Read the model definition and answer for the solid it produces. Units are mm, in the model's axes. A direction names the side the tool comes from. Give positions to 0.01 mm unless a question says otherwise; leave off trailing zeros. Write each loop counter-clockwise with the first axis right and the second up, starting at its lowest first coordinate (ties: lowest second). Pieces come first, ordered by that corner, then holes. Notation, with made-up numbers: M 54.25,-29 L 110.25,-29 A20 cw 110.25,-23 Z; hole C -24,30.5 d3. An arc over 180 degrees is marked long. Put each result on its own line as item: value.
from build123d import *

# Parameters (mm, degrees)
SKETCH1_W           = 230.12
SKETCH1_H           = 50.974909876
SKETCH1_R           = 7.058173785
BOSS_EXTRUDE1_DEPTH = 2
SKETCH2_R           = 10
BOSS_EXTRUDE2_DEPTH = 100
BOSS_EXTRUDE3_DEPTH = 10
FILLET1_R           = 5


with BuildPart() as part:
    # Sketch1 → Boss-Extrude1 (new body)
    with BuildSketch(Plane(origin=(0, 0, 0), x_dir=(1, 0, 0), z_dir=(0, 1, 0))):
        Rectangle(SKETCH1_W, SKETCH1_H)
        with Locations(Location((-95.06, 0, 0), (0, 0, 270))):
            Circle(SKETCH1_R, mode=Mode.SUBTRACT)
        with Locations(Location((95.06, 0, 0), (0, 0, 270))):
            Circle(SKETCH1_R, mode=Mode.SUBTRACT)
    extrude(amount=BOSS_EXTRUDE1_DEPTH)

    # Sketch2 → Boss-Extrude2 (add)
    with BuildSketch(Plane(origin=(0, 2, 0), x_dir=(1, 0, 0), z_dir=(0, 1, 0))):
        with Locations(Location((0, 0, 0), (0, 0, 270))):
            Circle(SKETCH2_R)
    extrude(amount=-BOSS_EXTRUDE2_DEPTH)

    # Sketch3 → Boss-Extrude3 (add)
    with BuildSketch(Plane(origin=(0, -98, 0), x_dir=(-1, 0, 0), z_dir=(0, -1, 0))):
        Polygon((15, 15), (30, 15), (30, -15), (15, -15), (15, -30), (-15, -30), (-15, -15), (-30, -15), (-30, 15), (-15, 15), (-15, 30), (15, 30), align=None)
    extrude(amount=BOSS_EXTRUDE3_DEPTH)

    # Fillet1
    fillet1_edges = [part.edges().sort_by_distance(p)[0] for p in [
        (0, 0, -10),
        (0, -98, -10),
    ]]
    fillet(fillet1_edges, radius=FILLET1_R)


solid = part.part
(1) Section A-A on z = 19.5 is taken. Determine the outline of the cut face in (x, y), and give its area (3 significant figures).
Result:
outline: M -115.06,0 L 115.06,0 L 115.06,2 L -115.06,2 Z; M -15,-108 L 15,-108 L 15,-98 L -15,-98 Z
area: 760 mm²
(2) Which of the six approach directions +Z, -Z, +X, -X, +Y, -Y give full straight-line access (tool end or side, diameter ignored) to faces 1 (the face through (-30, -103, 0)), 2 (the face through (-7, -98, -14)), 3 (the face through (23, -103, -15)), 4 (the face through (30, -103, 0)), 5 (the face through (22, -103, 15))?
Result:
face 1: +Z, -Z, -X, -Y
face 2: none
face 3: -Z, +X, -Y
face 4: +Z, -Z, +X, -Y
face 5: +Z, +X, -Y
(3) Section C-C on x = 95.06 is taken. Determine the outline of the cut face in (y, z).
Result:
outline: M 0,-25.49 L 2,-25.49 L 2,-7.06 L 0,-7.06 Z; M 0,7.06 L 2,7.06 L 2,25.49 L 0,25.49 Z
(4) Section D-D on x = 0 is taken. Determine the outline of the cut face in (y, z), and give its area (3 significant figures).
Result:
outline: M -108,-30 L -98,-30 L -98,-15 A5 cw -93,-10 L -5,-10 A5 cw 0,-15 L 0,-25.49 L 2,-25.49 L 2,25.49 L 0,25.49 L 0,15 A5 cw -5,10 L -93,10 A5 cw -98,15 L -98,30 L -108,30 Z
area: 2,680 mm²
(5) Given pin 1 Ø3 at (x, y) = (20.5, -103.5) entering from +Z; pin 2 Ø5 at (x, z) = (-53.5, -8) entering from -Y; pin 3 Ø11 at (y, z) = (-103, -21) entering from -X, each flat-ended and moving along its own axis, determine where each tip first touches the part or whether it passes through.
Result:
pin 1: stops at z = 15
pin 2: stops at y = 0
pin 3: stops at x = -15
(6) Straight lines are drawn through the part: line 1 along X through (y, z) = (0.9, 0); line 2 along Y through (x, z) = (56.5, -8); line 3 along Y through (x, z) = (-10.5, 26.5). For each, find the intervals that lie inside material, in ascending order. Write a range as from..to.
Result:
line 1: x = -115.06..-102.12, -88..88, 102.12..115.06
line 2: y = 0..2
line 3: y = -108..-98
(7) For a pull along Y with two mould halves and no side action, classify faces 6 (the face through (-15, -103, -23)), 7 (the face through (-2, 0, -17)), 8 (the face through (0, -108, 0)) as +Y half, -Y half, draft (parallel to the pull), parting line (faces both ways), or undercut.
Result:
face 6: draft
face 7: undercut
face 8: -Y half
(8) Section B-B on z = 0 is taken. Determine the outline of the cut face in (x, y).
Result:
outline: M -115.06,0 L -102.12,0 L -102.12,2 L -115.06,2 Z; M -88,0 L -15,0 A5 cw -10,-5 L -10,-93 A5 cw -15,-98 L -30,-98 L -30,-108 L 30,-108 L 30,-98 L 15,-98 A5 cw 10,-93 L 10,-5 A5 cw 15,0 L 88,0 L 88,2 L -88,2 Z; M 102.12,0 L 115.06,0 L 115.06,2 L 102.12,2 Z
